Autodesk Inventor part; units mm, degrees
ref_plane "YZ Plane" through (0, 0, 0) normal (1, 0, 0) x (0, 1, 0)
ref_plane "XZ Plane" through (0, 0, 0) normal (0, 1, 0) x (-1, 0, 0)
ref_plane "XY Plane" through (0, 0, 0) normal (0, 0, 1) x (1, 0, 0)
sketch "Sketch1" plane through (0, 0, 0) normal (0, 0, 1) x (1, 0, 0)
  line L0 (0, 25.4) -> (25.4, 25.4)
  line L1 (25.4, 25.4) -> (25.4, 76.2)
  line L2 (25.4, 76.2) -> (0, 76.2)
  line L3 (0, 76.2) -> (0, 25.4)
  line L4 (0, 25.4) -> (3.175, 25.4)
  line L5 (3.175, 25.4) -> (3.175, 28.575) construction
  line L6 (25.4, 76.2) -> (22.225, 76.2)
  line L7 (22.225, 76.2) -> (22.225, 73.025) construction
  line L8 (3.175, 28.575) -> (22.225, 28.575)
  line L9 (22.225, 28.575) -> (22.225, 73.025)
  line L10 (22.225, 73.025) -> (3.175, 73.025)
  line L11 (3.175, 73.025) -> (3.175, 28.575)
  point P0 (0, 0)
  dimension "d0" = 25.4
  dimension "d1" = 50.8
  dimension "d2" = 3.175
  dimension "d3" = 3.175
  dimension "d4" = 3.175
  dimension "d5" = 3.175
extrude "Extrusion1" add sketch "Sketch1" along normal blind 765.175
sketch "Sketch3" plane through (25.4, 25.4, 0) normal (1, 0, 0) x (0, 0, -1)
  line L0 (0, 0) -> (0, 50.8)
  line L1 (0, 50.8) -> (-765.175, 50.8)
  line L2 (-765.175, 0) -> (-765.175, 50.8)
  line L3 (0, 0) -> (-765.175, 0)
  line L4 (-765.175, 50.8) -> (-765.175, 0)
  line L5 (-765.175, 25.4) -> (-638.175, 25.4) construction
  circle A0 centre (-638.175, 25.4) radius 6.35
  point P0 (0, -25.4)
  dimension "d13" = 127
  dimension "d14" = 12.7
extrude "Extrusion3" cut sketch "Sketch3" against normal through all contours A0
sketch "Sketch4" plane through (0, 0, 0) normal (0, 0, -1) x (-1, 0, 0)
  line L0 (-3.175, 73.025) -> (-3.175, 28.575)
  line L1 (-3.175, 28.575) -> (-22.225, 28.575)
  line L2 (-22.225, 28.575) -> (-22.225, 73.025)
  line L3 (-22.225, 73.025) -> (-3.175, 73.025)
  line L4 (0, 25.4) -> (-25.4, 25.4)
  line L5 (0, 76.2) -> (0, 25.4)
  line L6 (-25.4, 76.2) -> (0, 76.2)
  line L7 (-25.4, 25.4) -> (-25.4, 76.2)
  point P0 (0, 0)
extrude "Extrusion4" add sketch "Sketch4" along normal blind 25.4
properties part number "ArmBar"
Work out the finished part from the listing and answer in its coordinate system (mm). A direction names the side the tool comes from. Give positions to 0.01 mm unless a question says otherwise; leave off trailing zeros. Write each loop counter-clockwise with the first axis right and the second up, starting at its lowest first coordinate (ties: lowest second). Pieces come first, ordered by that corner, then holes. Notation, with made-up numbers: (42, -9.75) - (60, -9.75) arc R18 cw to (60, -4.75) - close; hole circle Ø9 at (-11, 72.25). An arc over 180 degrees is marked (long way). One line per item, written item: value. Start each with the question number.
1. For faces 5 (the flat face through (13, 28.575, 375)), 6 (the flat face through (13, 25.4, 375)), determine the directions among +Z, -Z, +X, -X, +Y, -Y from which every point of the face is accessible in a straight line to the end or side of a thin tool.
2. Find section A-A (y = 50.8). Write down the section's boundary in (x, z) (3 decimals), then the cut area to 3 significant figures.
3. Find section C-C (z = 104). Write down the section's boundary in (x, y) (3 decimals), then the cut area to 3 significant figures.
4. Given pin 1 (7.5 mm diameter, centred on y = 50.8, z = 638.175, fed in from -X), flat-ended and moving along its own axis, determine where the tip first touches the part or whether it passes through.
5. Consider probe 1 along Y at (x, z) = (12, 340) (3 decimals); probe 2 along X at (y, z) = (41.5, 45) (3 decimals). Determine where each line is inside the solid, lowest interval first.
6. For a pull along X with two mould halves and no side action, classify faces 1 (the flat face through (22.225, 50, 375)), 2 (the flat face through (13, 73.025, 375)), 3 (the flat face through (25.4, 50, 375)), 4 (the flat face through (23, 49, -25.4)) as +X half, -X half, draft (parallel to the pull), parting line (faces both ways), or undercut.
7. Find section B-B (x = 18.25). Write down the section's boundary in (y, z) (3 decimals).
Geometry results:
1. face 5: +Z, -Z
1. face 6: +Z, -Z, +X, -X, -Y
2. outline: (0, -25.4) - (3.175, -25.4) - (3.175, 631.825) - (0, 631.825) - close; (0, 644.525) - (3.175, 644.525) - (3.175, 765.175) - (0, 765.175) - close; (22.225, -25.4) - (25.4, -25.4) - (25.4, 631.825) - (22.225, 631.825) - close; (22.225, 644.525) - (25.4, 644.525) - (25.4, 765.175) - (22.225, 765.175) - close
2. area: 4,940 mm2
3. outline: (0, 25.4) - (25.4, 25.4) - (25.4, 76.2) - (0, 76.2) - close; hole (3.175, 28.575) - (22.225, 28.575) - (22.225, 73.025) - (3.175, 73.025) - close
3. area: 444 mm2
4. pin 1: through
5. probe 1: 25.4 to 28.575, 73.025 to 76.2
5. probe 2: 0 to 3.175, 22.225 to 25.4
6. face 1: undercut
6. face 2: undercut
6. face 3: +X half
6. face 4: draft
7. outline: (25.4, -25.4) - (28.575, -25.4) - (28.575, 765.175) - (25.4, 765.175) - close; (73.025, -25.4) - (76.2, -25.4) - (76.2, 765.175) - (73.025, 765.175) - close
